```python
from build123d import *

# Parameters (mm, degrees)
EXTRUDE2_DEPTH     = 5
SKETCH3_W          = 1
SKETCH3_H          = 5
EXTRUDE3_DEPTH     = 10
CUT_EXTRUDE2_DEPTH = 5
EXTRUDE5_DEPTH     = 8
SKETCH8_W          = 1.5875
SKETCH8_H          = 5
EXTRUDE6_DEPTH     = 30
SKETCH9_W          = 1.5875
SKETCH9_H          = 30
EXTRUDE7_DEPTH     = 30
SKETCH10_W         = 1.5875
SKETCH10_H         = 30
EXTRUDE8_DEPTH     = 25
CUT_EXTRUDE3_DEPTH = 5
CUT_EXTRUDE4_DEPTH = 5
CUT_EXTRUDE6_DEPTH = 15
SKETCH15_R         = 0.7
CUT_EXTRUDE7_DEPTH = 10
EXTRUDE9_DEPTH     = 10
SKETCH18_R         = 1.5875
CUT_EXTRUDE8_DEPTH = 3
SKETCH19_R         = 1.5875
CUT_EXTRUDE9_DEPTH = 3


with BuildPart() as part:
    # Sketch2 → Extrude2 (new body)
    with BuildSketch(Plane.XY):
        with BuildLine():
            Line((-27.9875, 0), (-26.9875, 0))
            ThreePointArc((-26.9875, 0), (-19.083044257, 19.083044257), (0, 26.9875))
            ThreePointArc((0, 26.9875), (23.573172318, 17.223172318), (33.3375, -6.35))
            ThreePointArc((33.3375, -6.35), (19.853428439, -38.903428439), (-12.7, -52.3875))
            ThreePointArc((-12.7, -52.3875), (-58.72381262, -33.32381262), (-77.7875, 12.7))
            ThreePointArc((-77.7875, 12.7), (-51.284324863, 76.684324863), (12.7, 103.1875))
            ThreePointArc((12.7, 103.1875), (99.134965165, 67.384965165), (134.9375, -19.05))
            Line((134.9375, -19.05), (135.9375, -19.05))
            ThreePointArc((135.9375, -19.05), (99.842071946, 68.092071946), (12.7, 104.1875))
            ThreePointArc((12.7, 104.1875), (-51.991431644, 77.391431644), (-78.7875, 12.7))
            ThreePointArc((-78.7875, 12.7), (-59.430919402, -34.030919402), (-12.7, -53.3875))
            ThreePointArc((-12.7, -53.3875), (20.56053522, -39.61053522), (34.3375, -6.35))
            ThreePointArc((34.3375, -6.35), (24.280279099, 17.930279099), (0, 27.9875))
            ThreePointArc((0, 27.9875), (-19.790151038, 19.790151038), (-27.9875, 0))
        make_face()
    extrude(amount=EXTRUDE2_DEPTH)

    # Sketch3 → Extrude3 (add)
    with BuildSketch(Plane.XZ):
        with Locations((-27.4875, 2.5)):
            Rectangle(SKETCH3_W, SKETCH3_H)
    extrude(amount=EXTRUDE3_DEPTH)

    # Sketch6 → Cut-Extrude2 (cut)
    with BuildSketch(Plane(origin=(-26.9875, 0, 0), x_dir=(0, 0, -1), z_dir=(1, 0, 0))):
        Polygon((-5, -2.4), (-1.2, -10), (-5, -10), align=None)
    extrude(amount=-CUT_EXTRUDE2_DEPTH, mode=Mode.SUBTRACT)

    # Sketch7 → Extrude5 (add)
    with BuildSketch(Plane(origin=(-26.9875, 0, 0), x_dir=(0, 0, -1), z_dir=(1, 0, 0))):
        Polygon((-5, 0), (0, -10), (-1.2, -10), (-5, -2.4), align=None)
    extrude(amount=EXTRUDE5_DEPTH)

    # Sketch8 → Extrude6 (add)
    with BuildSketch(Plane.XZ.offset(19.05)):
        with Locations((135.73125, 2.5)):
            Rectangle(SKETCH8_W, SKETCH8_H)
    extrude(amount=EXTRUDE6_DEPTH)

    # Sketch9 → Extrude7 (add)
    with BuildSketch(Plane(origin=(0, 0, 0), x_dir=(-1, 0, 0), z_dir=(0, 0, -1))):
        with Locations((-135.73125, -34.05)):
            Rectangle(SKETCH9_W, SKETCH9_H)
    extrude(amount=EXTRUDE7_DEPTH)

    # Sketch10 → Extrude8 (add)
    with BuildSketch(Plane.XY.offset(5)):
        with Locations((135.73125, -34.05)):
            Rectangle(SKETCH10_W, SKETCH10_H)
    extrude(amount=EXTRUDE8_DEPTH)

    # Sketch11 → Cut-Extrude3 (cut)
    with BuildSketch(Plane.ZY.offset(-134.9375)):
        Polygon((5, -19.05), (30, -34.05), (30, -19.05), align=None)
    extrude(amount=-CUT_EXTRUDE3_DEPTH, mode=Mode.SUBTRACT)

    # Sketch12 → Cut-Extrude4 (cut)
    with BuildSketch(Plane.ZY.offset(-134.9375)):
        Polygon((5, -49.05), (-30, -29.728735128), (-30, -49.05), align=None)
    extrude(amount=-CUT_EXTRUDE4_DEPTH, mode=Mode.SUBTRACT)

    # Sketch14 → Cut-Extrude6 (cut)
    with BuildSketch(Plane.ZY.offset(27.9875)):
        Polygon((0, -5.5), (0, 14), (0.8, -5.5), (4.7625, -5.5), (4.7625, -10), (0, -10), align=None)
    extrude(amount=-CUT_EXTRUDE6_DEPTH, mode=Mode.SUBTRACT)

    # Sketch15 → Cut-Extrude7 (cut)
    with BuildSketch(Plane(origin=(0, -2, 4), x_dir=(-1, 0, 0), z_dir=(0, 0.447213595, -0.894427191))):
        with Locations((23.8125, -1)):
            Circle(SKETCH15_R)
        with Locations((20.6375, -1)):
            Circle(SKETCH15_R)
    extrude(amount=-CUT_EXTRUDE7_DEPTH, mode=Mode.SUBTRACT)

    # Sketch17 → Extrude9 (add)
    with BuildSketch(Plane(origin=(0, 0, -30), x_dir=(-1, 0, 0), z_dir=(0, 0, -1))):
        Polygon((-136.525, -19.05), (-136.525, -29.728735128), (-122.24, -65.09), (-120.65, -65.09), (-134.9375, -29.728735128), (-134.9375, -19.05), align=None)
    extrude(amount=EXTRUDE9_DEPTH)

    # Sketch18 → Cut-Extrude8 (cut)
    with BuildSketch(Plane(origin=(126.326271119, -51.041347224, 0), x_dir=(0, 0, 1), z_dir=(-0.927178193, 0.374620605, 0))):
        with Locations((-36.5125, -11.1125)):
            Circle(SKETCH18_R)
    extrude(amount=-CUT_EXTRUDE8_DEPTH, mode=Mode.SUBTRACT)

    # Sketch19 → Cut-Extrude9 (cut)
    with BuildSketch(Plane(origin=(136.525, 0, 0), x_dir=(0, 0, -1), z_dir=(1, 0, 0))):
        with Locations((-26.9875, -46.0375)):
            Circle(SKETCH19_R)
        with Locations((-26.9875, -36.5125)):
            Circle(SKETCH19_R)
        with Locations((-4.7625, -46.0375)):
            Circle(SKETCH19_R)
        with Locations((36.5125, -22.225)):
            Circle(SKETCH19_R)
    extrude(amount=-CUT_EXTRUDE9_DEPTH, mode=Mode.SUBTRACT)


solid = part.part
```
Design review of the part built by this model. Coordinates are the model's own, in mm. A direction names the side the tool comes from. Give positions to 0.01 mm unless a question says otherwise; leave off trailing zeros. Order: outer loops, then holes, each group sorted by start corner. A loop starts at its lowest first (then second) coordinate and runs counter-clockwise, first axis right, second up. Notation, with made-up numbers: (57, 34) - (108, 34) arc R37 cw to (108, 73) - close; hole circle Ø10 at (-26.75, 19.5). An arc over 180 degrees is marked (long way). Use a Markdown table: item, result. Add a question column.
(1) Add section A-A on x = 16.5. Give the boundary of the cut face in (y, z), then the cut area to 3 significant figures.
(2) Mouldability with a two-part tool opening along X and no side actions: class faces 1 (the face through (130.4, -42, -40)), 2 (the face through (-51.98, 75.98, 2.46)), 3 (the face through (-59.942, -33.514, 2.465)), 4 (the face through (129.482, -47.162, -34.93)) as +X half, -X half, draft (parallel to the pull), parting line (faces both ways), or undercut.
(3) Add section C-C on x = -35.5. Give the boundary of the cut face in (y, z).
(4) Machinability: for faces 5 (the face through (-23, -2, 4)), 6 (the face through (-51.276, 78.099, 2.465)), 7 (the face through (-19.57, 20.01, 2.46)), 8 (the face through (20.193, -39.974, 2.465)), which of the approach directions +Z, -Z, +X, -X, +Y, -Y give a long, thin tool a straight path to every point of the face, cutting with its end or side? Answer none if there is none.
(5) Wall thickness on probe 1 along Z at (x, y) = (-13.5, 24); probe 2 along X at (y, z) = (-46, 22.5) (1 decimal); probe 3 along Y at (x, z) = (127.5, -33): over which ranges is each line inside the solid? List them lowest first. Write a range as [from, to].
(6) Clearance check with flat-ended pins moving along their axes: P1, Ø2.5, axis at y = -46.04, z = 26.99, coming from the -X side; P2, Ø5, axis at y = -2, z = 2.5, coming from the -X side; P3, Ø2, axis at y = -2, z = 3, coming from the +X side; P4, Ø12, axis at x = 112, z = 8.5, coming from the +Y side. State where each tip first meets the part, or that it passes through.
Report:
| question | item | result |
|---|---|---|
| 1 | outline | (-43.23, 0) - (-41.94, 0) - (-41.94, 5) - (-43.23, 5) - close; (22.62, 0) - (23.76, 0) - (23.76, 5) - (22.62, 5) - close; (103.13, 0) - (104.13, 0) - (104.13, 5) - (103.13, 5) - close |
| 1 | area | 17.2 mm² |
| 2 | face 1 | draft |
| 2 | face 2 | undercut |
| 2 | face 3 | -X half |
| 2 | face 4 | +X half |
| 3 | outline | (-49.33, 0) - (-48.26, 0) - (-48.26, 5) - (-49.33, 5) - close; (89.28, 0) - (90.46, 0) - (90.46, 5) - (89.28, 5) - close |
| 4 | face 5 | -Z |
| 4 | face 6 | +Z, -Z, -X, +Y |
| 4 | face 7 | +Z, -Z |
| 4 | face 8 | +Z, -Z, -Y |
| 5 | probe 1 | z = [0, 5] |
| 5 | probe 2 | x = [134.9, 136.5] |
| 5 | probe 3 | y = [-52.07, -48.14] |
| 6 | P1 | passes through |
| 6 | P2 | stops at x = -77.65 |
| 6 | P3 | stops at x = 134.89 |
| 6 | P4 | stops at y = 60.14 |
